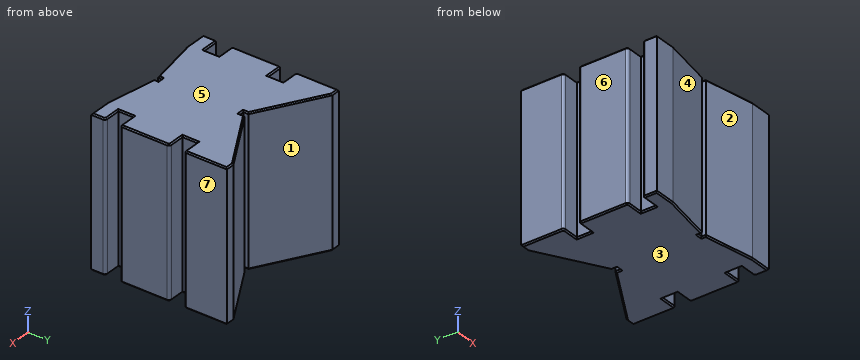
```python
from build123d import *

# Parameters (mm, degrees)
BOSS_EXTRUDE1_DEPTH = 60
SKETCH3_W           = 2
SKETCH3_H           = 3
CUT_EXTRUDE1_DEPTH  = 73.601820229
CHAMFER1_SIZE       = 0.5


with BuildPart() as part:
    # Sketch1 → Boss-Extrude1 (new body)
    with BuildSketch(Plane.XY):
        with BuildLine():
            Line((-30, 0), (-30, 3))
            ThreePointArc((-30, 3), (-29.707106781, 3.707106781), (-29, 4))
            Line((-29, 4), (-23, 4))
            Line((-23, 4), (-23, 10))
            Line((-23, 10), (-29, 10))
            ThreePointArc((-29, 10), (-29.707106781, 10.292893219), (-30, 11))
            Line((-30, 11), (-30, 27.299782134))
            Line((-30, 27.299782134), (-26.5, 27.299782134))
            Line((-26.5, 27.299782134), (0, 12))
            Line((0, 12), (26.5, 27.299782134))
            Line((26.5, 27.299782134), (30, 27.299782134))
            Line((30, 27.299782134), (30, 11))
            ThreePointArc((30, 11), (29.707106781, 10.292893219), (29, 10))
            Line((29, 10), (23, 10))
            Line((23, 10), (23, 4))
            Line((23, 4), (29, 4))
            ThreePointArc((29, 4), (29.707106781, 3.707106781), (30, 3))
            Line((30, 3), (30, 0))
            Line((30, 0), (30, -15))
            ThreePointArc((30, -15), (29.707106781, -15.707106781), (29, -16))
            Line((29, -16), (23, -16))
            Line((23, -16), (23, -22))
            Line((23, -22), (29, -22))
            ThreePointArc((29, -22), (29.707106781, -22.292893219), (30, -23))
            Line((30, -23), (30, -27.767324332))
            Line((30, -27.767324332), (21.36555799, -27.767324332))
            Line((21.36555799, -27.767324332), (0, -24))
            Line((0, -24), (-21.36555799, -27.767324332))
            Line((-21.36555799, -27.767324332), (-30, -27.767324332))
            Line((-30, -27.767324332), (-30, -23))
            ThreePointArc((-30, -23), (-29.707106781, -22.292893219), (-29, -22))
            Line((-29, -22), (-23, -22))
            Line((-23, -22), (-23, -16))
            Line((-23, -16), (-29, -16))
            ThreePointArc((-29, -16), (-29.707106781, -15.707106781), (-30, -15))
            Line((-30, -15), (-30, 0))
        make_face()
    extrude(amount=BOSS_EXTRUDE1_DEPTH)

    # Sketch3 → Cut-Extrude1 (cut, through all)
    with BuildSketch(Plane(origin=(0, 0, 0), x_dir=(-1, 0, 0), z_dir=(0, 0, -1))):
        with Locations((0, 12)):
            Rectangle(SKETCH3_W, SKETCH3_H)
        with Locations((0, -24)):
            Rectangle(SKETCH3_W, SKETCH3_H)
    extrude(amount=-CUT_EXTRUDE1_DEPTH, mode=Mode.SUBTRACT)

    # Chamfer1
    chamfer1_edges = [part.edges().sort_by_distance(p)[0] for p in [
        (-29.707106781, 3.707106781, 60),
        (-26, 4, 60),
        (-23, 7, 60),
        (-26, 10, 60),
        (-29.707106781, 10.292893219, 60),
        (-30, 19.149891067, 60),
        (-28.25, 27.299782134, 60),
        (-13.75, 19.938566201, 60),
        (13.75, 19.938566201, 60),
        (28.25, 27.299782134, 60),
        (30, 19.149891067, 60),
        (29.707106781, 10.292893219, 60),
        (26, 10, 60),
        (23, 7, 60),
        (26, 4, 60),
        (29.707106781, 3.707106781, 60),
        (30, -6, 60),
        (29.707106781, -15.707106781, 60),
        (26, -16, 60),
        (23, -19, 60),
        (26, -22, 60),
        (29.707106781, -22.292893219, 60),
        (30, -25.383662166, 60),
        (25.682778995, -27.767324332, 60),
        (11.182778995, -25.971825656, 60),
        (-11.182778995, -25.971825656, 60),
        (-25.682778995, -27.767324332, 60),
        (-30, -25.383662166, 60),
        (-29.707106781, -22.292893219, 60),
        (-26, -22, 60),
        (-23, -19, 60),
        (-26, -16, 60),
        (-29.707106781, -15.707106781, 60),
        (-30, -6, 60),
        (-26, -16, 0),
        (-23, -19, 0),
        (-26, -22, 0),
        (-29.707106781, -22.292893219, 0),
        (-30, -25.383662166, 0),
        (-25.682778995, -27.767324332, 0),
        (-11.182778995, -25.971825656, 0),
        (11.182778995, -25.971825656, 0),
        (25.682778995, -27.767324332, 0),
        (30, -25.383662166, 0),
        (29.707106781, -22.292893219, 0),
        (26, -22, 0),
        (23, -19, 0),
        (26, -16, 0),
        (29.707106781, -15.707106781, 0),
        (30, -6, 0),
        (29.707106781, 3.707106781, 0),
        (26, 4, 0),
        (23, 7, 0),
        (26, 10, 0),
        (29.707106781, 10.292893219, 0),
        (30, 19.149891067, 0),
        (28.25, 27.299782134, 0),
        (13.75, 19.938566201, 0),
        (-13.75, 19.938566201, 0),
        (-28.25, 27.299782134, 0),
        (-30, 19.149891067, 0),
        (-29.707106781, 10.292893219, 0),
        (-26, 10, 0),
        (-23, 7, 0),
        (-26, 4, 0),
        (-29.707106781, 3.707106781, 0),
        (-30, -6, 0),
        (-29.707106781, -15.707106781, 0),
        (1, -23.33816349, 60),
        (0, -22.5, 60),
        (-1, -23.33816349, 60),
        (-1, 11.538675135, 60),
        (0, 10.5, 60),
        (1, 11.538675135, 60),
        (-1, 11.538675135, 0),
        (-1, -23.33816349, 0),
        (0, -22.5, 0),
        (1, -23.33816349, 0),
        (1, 11.538675135, 0),
        (0, 10.5, 0),
    ]]
    chamfer(chamfer1_edges, length=CHAMFER1_SIZE)


solid = part.part
```
Model file for the job. Use its own axes, mm. Face numbers are marked on the shaded views. A direction names the side the tool comes from. Coordinates: 2 decimals unless noted, no trailing zeros. Loops run counter-clockwise (first coordinate to the right, second up) from the corner with the lowest first, then second, coordinate; pieces in that order, holes last. Notation, with made-up numbers: (47.5, 4) - (71.5, 4) arc R19 cw to (71.5, 25) - close; hole circle Ø3 at (-5, -13). An arc over 180 degrees is marked (long way). Write item = value, one per line. Start each with the question number.
Item 1: 3-axis set-ups, long thin cutter, end or side, ignore diameter. For the marked faces 1, 2 and 3: which of +Z, -Z, +X, -X, +Y, -Y reach the whole face in a straight line?
Item 2: Pull direction X, two halves, no side cores. Call the marked faces 4, 5, 6 and 7: +X half, -X half, draft (parallel to the pull), parting line (faces both ways), or undercut.
Item 3: Saw through at B-B, the plane x = 24. List the corners of the cut face in (y, z).
Item 4: Saw through at C-C, the plane x = -15. List the corners of the cut face in (y, z).
Item 5: Drop flat-ended pins along their axis: pin 1 Ø12 at (x, z) = (-15, 47) entering from +Y; pin 2 Ø6.5 at (y, z) = (-19, 33.5) entering from -X; pin 3 Ø5 at (x, z) = (10, 29.5) entering from +Y. Give the stop position or say it passes through.
Item 6: Saw through at D-D, the plane y = 17. List the corners of the cut face in (x, z).
Item 7: Saw through at A-A, the plane y = 23.5. List the corners of the cut face in (x, z).
Item 8: Wall check: probe 1 along Y at (x, z) = (-24, 30); probe 2 along Y at (x, z) = (23.5, 19.5); probe 3 along X at (y, z) = (13.5, 13). Give the ranges that are in metal, low to high. Write a range as [from, to].
Answers:
q1.face_1 = +Z, -Z, +Y
q1.face_2 = +Z, -Z, -Y
q1.face_3 = -Z, +X, -X, +Y, -Y
q2.face_4 = undercut
q2.face_5 = draft
q2.face_6 = -X half
q2.face_7 = +X half
q3.outline = (-27.77, 0.5) - (-27.27, 0) - (-22.5, 0) - (-22, 0.5) - (-22, 59.5) - (-22.5, 60) - (-27.27, 60) - (-27.77, 59.5) - close; (-16, 0.5) - (-15.5, 0) - (3.5, 0) - (4, 0.5) - (4, 59.5) - (3.5, 60) - (-15.5, 60) - (-16, 59.5) - close; (10, 0.5) - (10.5, 0) - (25.28, 0) - (25.86, 0.5) - (25.86, 59.5) - (25.28, 60) - (10.5, 60) - (10, 59.5) - close
q4.outline = (-26.64, 0.5) - (-26.14, 0) - (20.08, 0) - (20.66, 0.5) - (20.66, 59.5) - (20.08, 60) - (-26.14, 60) - (-26.64, 59.5) - close
q5.pin_1 = 24.12
q5.pin_2 = -29.66
q5.pin_3 = 19.22
q6.outline = (-30, 0.5) - (-29.5, 0) - (-9.66, 0) - (-8.66, 0.5) - (-8.66, 59.5) - (-9.66, 60) - (-29.5, 60) - (-30, 59.5) - close; (8.66, 0.5) - (9.66, 0) - (29.5, 0) - (30, 0.5) - (30, 59.5) - (29.5, 60) - (9.66, 60) - (8.66, 59.5) - close
q7.outline = (-30, 0.5) - (-29.5, 0) - (-20.92, 0) - (-19.92, 0.5) - (-19.92, 59.5) - (-20.92, 60) - (-29.5, 60) - (-30, 59.5) - close; (19.92, 0.5) - (20.92, 0) - (29.5, 0) - (30, 0.5) - (30, 59.5) - (29.5, 60) - (20.92, 60) - (19.92, 59.5) - close
q8.probe_1 = [-27.77, -22], [-16, 4], [10, 25.86]
q8.probe_2 = [-27.77, -22], [-16, 4], [10, 25.57]
q8.probe_3 = [-30, -2.6], [2.6, 30]
